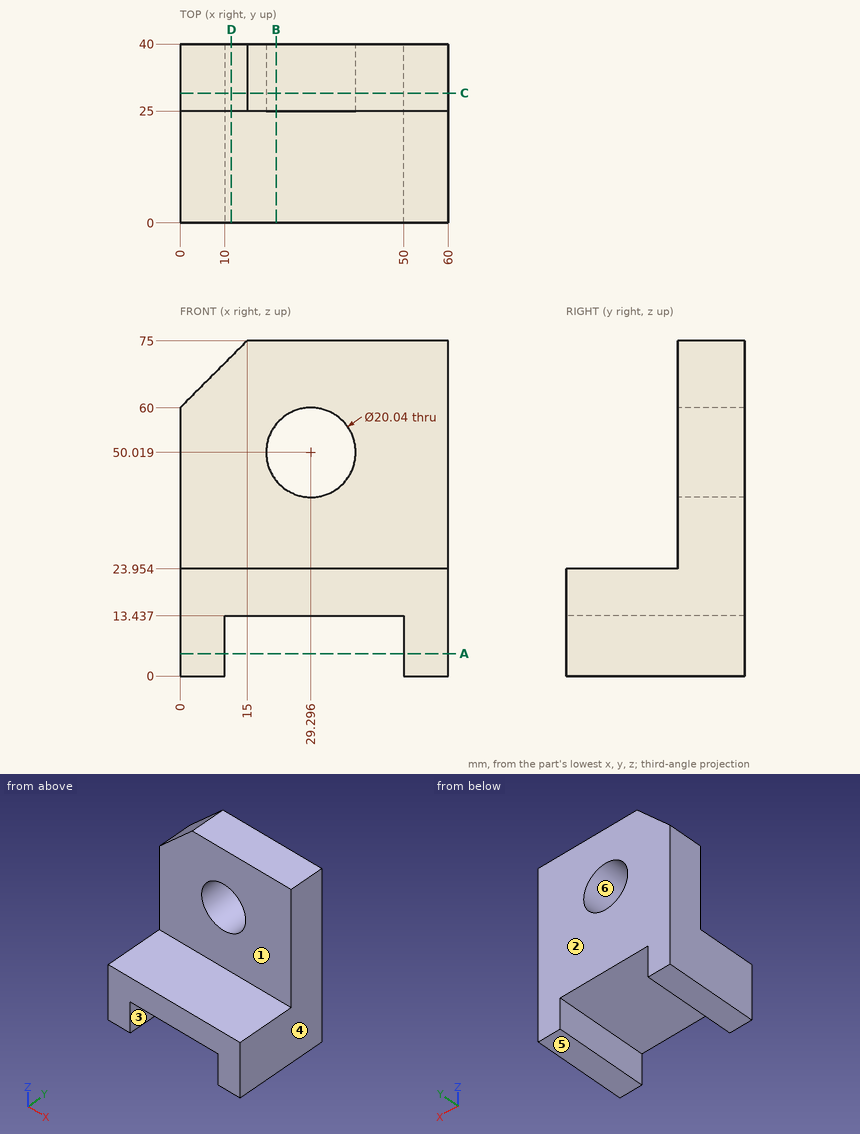
Input: dimensioned drawing with shaded views. Units: mm. Origin: part minimum x, y, z. A direction names the side the tool comes from. Give positions to 0.01 mm unless a question says otherwise; leave off trailing zeros. Loops run counter-clockwise (first coordinate to the right, second up) from the corner with the lowest first, then second, coordinate; pieces in that order, holes last. Notation, with made-up numbers: M -33,-4 L -5,-4 A17 cw -5,7 Z; hole C 18,-20.5 d11. An arc over 180 degrees is marked long. Put each result on its own line as item: value. Start each with the question number.
1) Ray query, line 1 along X through (y, z) = (26, 4); line 2 along Z through (x, y) = (57, 14.5) (1 decimal); line 3 along Y through (x, z) = (16.5, 69). Return the intervals inside material, ascending.
2) Cut plane B-B (x = 21.5). Output: boundary loops of the cut face in (y, z) (1 decimal).
3) Cut plane D-D (x = 11.5). Output: boundary loops of the cut face in (y, z) (1 decimal).
4) Contact query for flat-ended pins moving along their axis: pin 1 (3 mm diameter, centred on x = 49, y = 15, fed in from +Z); pin 2 (15.5 mm diameter, centred on x = 31, z = 56.5, fed in from -Y); pin 3 (12 mm diameter, centred on x = 21, y = 17, fed in from -Z). Output: stop coordinate, or through.
5) Access query for the marked faces 1, 2 and 3. Directions: +Z, -Z, +X, -X, +Y, -Y. A direction counts if a zero-diameter tool reaches every point of the face in a straight line with its end or side. Return the directions, or none.
6) Cut plane C-C (y = 29). Output: boundary loops of the cut face in (x, z).
7) Cut plane A-A (z = 5). Output: boundary loops of the cut face in (x, y), then the cut area to 3 significant figures.
8) Pull-direction query (X, two-part tool) for the marked faces 4, 5 and 6; classes: pulls with the +X half, pulls with the -X half, needs draft (parallel to the pull), parting line crosses it, or undercut.
Verdict:
1. line 1: 0 to 10, 50 to 60
1. line 2: 0 to 24
1. line 3: 25 to 40
2. outline: M 0,13.4 L 40,13.4 L 40,43.7 L 25,43.7 L 25,24 L 0,24 Z; M 25,56.3 L 40,56.3 L 40,75 L 25,75 Z
3. outline: M 0,13.4 L 40,13.4 L 40,71.5 L 25,71.5 L 25,24 L 0,24 Z
4. pin 1: z = 23.95
4. pin 2: y = 25
4. pin 3: z = 13.44
5. face 1: +Z, +X, -X, -Y
5. face 2: +Z, -Z, +X, -X, +Y
5. face 3: -Z, +Y, -Y
6. outline: M 0,0 L 10,0 L 10,13.44 L 50,13.44 L 50,0 L 60,0 L 60,75 L 15,75 L 0,60 Z; hole C 29.3,50.02 d20.04
7. outline: M 0,0 L 10,0 L 10,40 L 0,40 Z; M 50,0 L 60,0 L 60,40 L 50,40 Z
7. area: 800 mm2
8. face 4: pulls with the +X half
8. face 5: needs draft
8. face 6: undercut
